CAD build for the part. Positions are in the model's coordinates, mm. Face numbers are marked on the shaded views. A direction names the side the tool comes from. Give positions to 0.01 mm unless a question says otherwise; leave off trailing zeros. Loops run counter-clockwise (first coordinate to the right, second up) from the corner with the lowest first, then second, coordinate; pieces in that order, holes last.
Item 1: Probe probe 1 along Z at (x, y) = (0.5, 8); probe 2 along X at (y, z) = (4.25, -24.13); probe 3 along X at (y, z) = (8.5, 28) (1 decimal). List the from-to ranges inside material, lowest first.
Item 2: Drop flat-ended pins along their axis: P1, Ø2, axis at x = 0.4, y = 6.49, coming from the +Z side; P2, Ø5, axis at x = 3.5, y = 2, coming from the +Z side; P3, Ø6, axis at x = 2, y = 7.5, coming from the +Z side. Give the stop position or say it passes through.
Item 3: Saw through at D-D on z = 41.5. Give the cut face in (x, y), plus the area to 3 significant figures.
Item 4: Which spindle directions (+Z, -Z, +X, -X, +Y, -Y) get a long thin tool onto all of the face, cutting with end or side? Do the marked faces 1 and 2. Say none if no direction does.
Item 5: Mould opens along X. For the marked faces 3, 4, 5 and 6 say: released by +X, released by -X, zero draft, split by the parting line, or undercut.
Item 6: Saw through at A-A on z = -24.13. Give the cut face in (x, y).
Item 7: Saw through at B-B on y = 11.75. Give the number of separate pieces and of enclosed holes in the cut face, plus the area to 3 significant figures.
Autodesk Inventor part; units mm, degrees
ref_plane "YZ Plane" through (0, 0, 0) normal (1, 0, 0) x (0, 1, 0)
ref_plane "XZ Plane" through (0, 0, 0) normal (0, 1, 0) x (-1, 0, 0)
ref_plane "XY Plane" through (0, 0, 0) normal (0, 0, 1) x (1, 0, 0)
sketch "Sketch1" plane through (0, 0, 0) normal (0, 1, 0) x (-1, 0, 0)
  line L0 (-9.2075, -46.99) -> (9.2075, -46.99)
  line L1 (15.5575, -40.64) -> (15.5575, 46.99)
  line L2 (-15.5575, 46.99) -> (-15.5575, -40.64)
  line L3 (-15.5575, -46.99) -> (15.5575, 46.99) construction
  line L4 (15.5575, -46.99) -> (-15.5575, 46.99) construction
  circle A0 centre (0, -24.13) radius 6.35
  line L5 (9.525, -6.6675) -> (9.525, 29.21)
  line L6 (-9.525, 29.21) -> (-9.525, -6.6675)
  line L7 (-9.525, -6.6675) -> (9.525, 29.21) construction
  line L8 (9.525, -6.6675) -> (-9.525, 29.21) construction
  arc A1 (9.525, 29.21) -> (-9.525, 29.21) centre (0, 29.21) ccw
  arc A2 (-9.525, -6.6675) -> (9.525, -6.6675) centre (0, -6.6675) ccw
  line L9 (-8.89, 46.99) -> (-15.5575, 46.99)
  arc A3 (9.2075, -46.99) -> (15.5575, -40.64) centre (9.2075, -40.64) ccw
  arc A4 (-15.5575, -40.64) -> (-9.2075, -46.99) centre (-9.2075, -40.64) ccw
  line L10 (0, 71.5612) -> (0, -73.6541)
  arc A5 (-8.9803, 46.99) -> (8.9803, 46.99) centre (0, 50.165) ccw
  line L11 (15.5575, 46.99) -> (8.9803, 46.99)
  line L12 (-8.9803, 46.99) -> (-15.5575, 46.99)
  point P0 (0, 0)
  point P1 (0, 11.2712)
  point P2 (0, 0)
  point P3 (0, 11.2712)
  dimension "d0" = 93.98
  dimension "d1" = 31.115
  dimension "d2" = 22.86
  dimension "d3" = 12.7
  dimension "d4" = 35.8775
  dimension "d5" = 19.05
  dimension "d7" = 6.35
  dimension "d12" = 19.05
  dimension "d13" = 17.78
  dimension "d14" = 3.175
extrude "Extrusion1" add sketch "Sketch1" along normal blind 12.7 contours A4 L2 L9 A5 L10 A1 L6 A2 A0 L0 | L10 A0 A2 L5 A1 A5 L11 L1 A3 L0
sketch "Sketch3" plane through (8.9803, 0, 46.99) normal (0, 0, 1) x (1, 0, 0)
  line L0 (-24.5378, 0) -> (-17.9605, 0)
  line L1 (-17.9605, 0) -> (-17.9605, 3.048)
  line L2 (-17.9605, 3.048) -> (-24.5378, 3.048)
  line L3 (-24.5378, 3.048) -> (-24.5378, 0)
  line L4 (6.5772, 0) -> (0, 0)
  line L5 (0, 0) -> (0, 3.048)
  line L6 (0, 3.048) -> (6.5772, 3.048)
  line L7 (6.5772, 3.048) -> (6.5772, 0)
  point P0 (-8.9803, 0)
  point P1 (0, 12.7)
  point P2 (-17.9605, 12.7)
  dimension "d15" = 3.048
extrude "Extrusion2" add sketch "Sketch3" along normal blind 1.524
hole "Hole1" at (0.3982, 6.4915, -46.99) direction (0, 0, 1) diameter 2.6416 depth 17.78 tip angle 118
equation "\"d12\" = d5"
properties part number "Fixture_Slide_Lock_Plate"
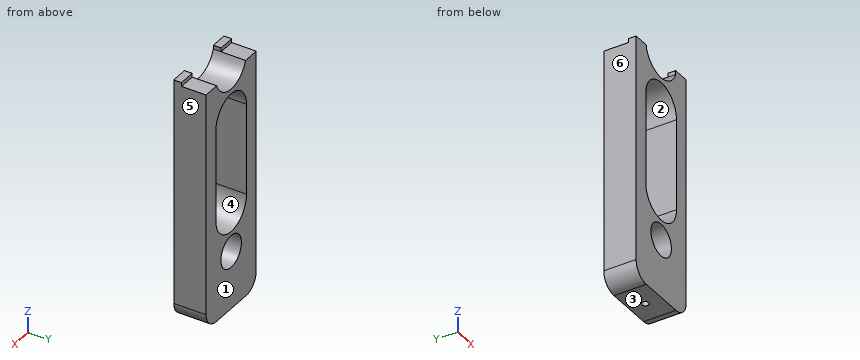
Results below:
1. probe 1: z = -46.99 to -30.46, -17.8 to -16.18, 38.72 to 40.65
1. probe 2: x = -15.56 to -6.35, 6.35 to 15.56
1. probe 3: x = -15.6 to -9.5, 9.5 to 15.6
2. P1: stops at z = 40.74
2. P2: stops at z = 42.77
2. P3: stops at z = 42.06
3. outline: (-15.56, 0) - (-3.96, 0) - (-3.96, 12.7) - (-15.56, 12.7) - close; (3.96, 0) - (15.56, 0) - (15.56, 12.7) - (3.96, 12.7) - close
3. area: 295 mm2
4. face 1: +Z, -Z, +X, -X, +Y
4. face 2: +Y, -Y
5. face 3: zero draft
5. face 4: undercut
5. face 5: released by +X
5. face 6: released by -X
6. outline: (-15.56, 0) - (-6.35, 0) - (-6.35, 12.7) - (-15.56, 12.7) - close; (6.35, 0) - (15.56, 0) - (15.56, 12.7) - (6.35, 12.7) - close
7. separate pieces: 1
7. enclosed holes: 2
7. area: 1,730 mm2
